```python
from build123d import *

# Parameters (mm, degrees)
BOSS_EXTRUDE1_DEPTH      = 12.7
SKETCH2_R                = 2.25
CUT_EXTRUDE1_DEPTH       = 12.7
BOSS_EXTRUDE4_DEPTH      = 12.7
SKETCH4_R                = 20.25
CUT_EXTRUDE2_DEPTH       = 2
SKETCH6_R                = 20.325
BOSS_EXTRUDE5_DEPTH      = 1.5
SKETCH5_R                = 9.53
CUT_EXTRUDE3_DEPTH       = 30
SKETCH8_W                = 6.62
SKETCH8_H                = 12.7
BOSS_EXTRUDE7_DEPTH      = 3.1
BOSS_EXTRUDE7_DEPTH_BACK = 6.2


with BuildPart() as part:
    # Sketch1 → Boss-Extrude1 (new body)
    with BuildSketch(Plane.XY):
        Polygon((0, 21), (21, 21), (21, -21), (-21, -21), (-21, 21), align=None)
    extrude(amount=BOSS_EXTRUDE1_DEPTH)

    # Sketch2 → Cut-Extrude1 (cut)
    with BuildSketch(Plane.XY):
        with Locations((17.500892834, 17.500892834)):
            Circle(SKETCH2_R)
        with Locations((-17.500892834, -17.500892834)):
            Circle(SKETCH2_R)
    extrude(amount=CUT_EXTRUDE1_DEPTH, mode=Mode.SUBTRACT)

    # Sketch3 → Boss-Extrude4 (add)
    with BuildSketch(Plane.XY.offset(12.7)):
        with BuildLine():
            Line((-21, -12.460892834), (-27.5, -12.460892834))
            Line((-27.5, -12.460892834), (-27.5, -13.160892834))
            Line((-27.5, -13.160892834), (-28.57, -13.160892834))
            Line((-28.57, -13.160892834), (-28.57, -9.240892834))
            add(Edge.make_bspline(
                [(-28.57, 9.240892834), (-36.45, 0), (-28.57, -9.240892834)],
                knots=[0, 0, 0, 1, 1, 1], degree=2))
            Line((-28.57, 9.240892834), (-28.57, 13.160892834))
            Line((-28.57, 13.160892834), (-27.5, 13.160892834))
            Line((-27.5, 13.160892834), (-27.5, 12.460892834))
            Line((-27.5, 12.460892834), (-21, 12.460892834))
            Line((-21, 12.460892834), (-21, -12.460892834))
        make_face()
    extrude(amount=-BOSS_EXTRUDE4_DEPTH)

    # Sketch4 → Cut-Extrude2 (cut)
    with BuildSketch(Plane.XY.offset(12.7)):
        Circle(SKETCH4_R)
    extrude(amount=-CUT_EXTRUDE2_DEPTH, mode=Mode.SUBTRACT)

    # Sketch6 → Boss-Extrude5 (add)
    with BuildSketch(Plane(origin=(0, 0, 0), x_dir=(-1, 0, 0), z_dir=(0, 0, -1))):
        Circle(SKETCH6_R)
    extrude(amount=BOSS_EXTRUDE5_DEPTH)

    # Sketch5 → Cut-Extrude3 (cut)
    with BuildSketch(Plane.XY.offset(10.7)):
        Circle(SKETCH5_R)
    extrude(amount=-CUT_EXTRUDE3_DEPTH, mode=Mode.SUBTRACT)

    # Sketch8 → Boss-Extrude7 (add, two sides)
    with BuildSketch(Plane.XY.offset(12.7)) as boss_extrude7_sk:
        with Locations((-31.88, 0.210892834)):
            Rectangle(SKETCH8_W, SKETCH8_H)
    extrude(amount=BOSS_EXTRUDE7_DEPTH)
    extrude(boss_extrude7_sk.sketch, amount=-BOSS_EXTRUDE7_DEPTH_BACK)


solid = part.part
```
Verification items for the finished model (mm, model axes). A direction names the side the tool comes from. Round coordinates to 2 decimals unless told otherwise and drop trailing zeros. Write each loop counter-clockwise with the first axis right and the second up, starting at its lowest first coordinate (ties: lowest second). Pieces come first, ordered by that corner, then holes.
1. Section check A-A on x = 0. Enter the section's corners in (y, z) (3 decimals).
2. Section check D-D on x = 12. Enter the section's corners in (y, z), plus the area to 3 significant figures.
3. Gauge pin test, flat ends, axial feed: P1, Ø2.5, axis at y = 18.5, z = 6.5, coming from the -X side; P2, Ø0.5, axis at x = -28, z = 6.5, coming from the -Y side; P3, Ø12.5, axis at x = -13.5, y = -10.5, coming from the +Z side. Record the tip position at first contact, or that the pin passes through.
4. Access from +Z, -Z, +X, -X, +Y, -Y to the whole of each face (thin tool, end or side, straight path). Record for faces 1 (the flat face through (-33, -6.139, 11)), 2 (the flat face through (-24, 12.461, 6)), 3 (the flat face through (-33, 6.561, 11)), 4 (the flat face through (-20.4, 3.2, 0)).
5. Section check B-B on x = 6. Enter the section's corners in (y, z).
6. Draft check along Y on faces 5 (the flat face through (-4, -9, -1.5)), 6 (the flat face through (0, -21, 6)), 7 (the cylindrical face through (-1.24, 9.45, 4.69)). Enter one of: +Y half, -Y half, draft (parallel to the pull), parting line (faces both ways), or undercut.
7. Scan lines: L1, parallel to Y at x = 0, z = 1.75; L2, parallel to Z at x = 7.5, y = -14.5; L3, parallel to X at y = 16.5, z = 7.5. Record each from-to range of solid material in increasing order.
8. Section check C-C on z = 15. Enter the section's corners in (x, y).
Answer:
1. outline: (-21, 0) - (-20.325, 0) - (-20.325, -1.5) - (-9.53, -1.5) - (-9.53, 10.7) - (-20.25, 10.7) - (-20.25, 12.7) - (-21, 12.7) - close; (9.53, -1.5) - (20.325, -1.5) - (20.325, 0) - (21, 0) - (21, 12.7) - (20.25, 12.7) - (20.25, 10.7) - (9.53, 10.7) - close
2. outline: (-21, 0) - (-16.4, 0) - (-16.4, -1.5) - (16.4, -1.5) - (16.4, 0) - (21, 0) - (21, 12.7) - (16.31, 12.7) - (16.31, 10.7) - (-16.31, 10.7) - (-16.31, 12.7) - (-21, 12.7) - close
2. area: 517 mm2
3. P1: stops at x = -21
3. P2: stops at y = -13.16
3. P3: stops at z = 12.7
4. face 1: +Z, -X, -Y
4. face 2: +Z, -Z, +Y
4. face 3: +Z, -X, +Y
4. face 4: -Z
5. outline: (-21, 0) - (-19.42, 0) - (-19.42, -1.5) - (-7.4, -1.5) - (-7.4, 10.7) - (-19.34, 10.7) - (-19.34, 12.7) - (-21, 12.7) - close; (7.4, -1.5) - (19.42, -1.5) - (19.42, 0) - (21, 0) - (21, 12.7) - (19.34, 12.7) - (19.34, 10.7) - (7.4, 10.7) - close
6. face 5: draft
6. face 6: -Y half
6. face 7: undercut
7. L1: y = -21 to -9.53, 9.53 to 21
7. L2: z = -1.5 to 10.7
7. L3: x = -21 to 15.49, 19.52 to 21
8. outline: (-35.19, -6.14) - (-28.57, -6.14) - (-28.57, 6.56) - (-35.19, 6.56) - close
